Can you work these out from the model? Positions are in its coordinate system, mm. Face numbers are marked on the shaded views. A direction names the side the tool comes from. Coordinates: 2 decimals unless noted, no trailing zeros. Loops run counter-clockwise (first coordinate to the right, second up) from the corner with the lowest first, then second, coordinate; pieces in that order, holes last.
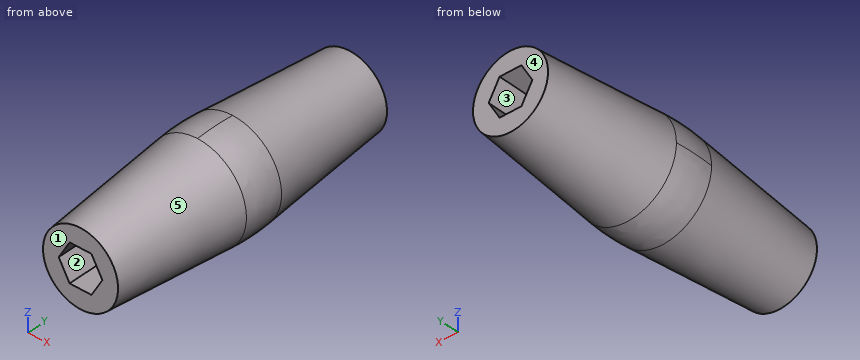
```python
from build123d import *

# Parameters (mm, degrees)
SKETCH1_R           = 12.7
BOSS_EXTRUDE1_DEPTH = 101.6
SKETCH2_R           = 12.7
BOSS_EXTRUDE2_DEPTH = 50.8
BOSS_EXTRUDE2_DRAFT = 5
SKETCH3_R           = 12.7
BOSS_EXTRUDE3_DEPTH = 50.8
BOSS_EXTRUDE3_DRAFT = 5
CUT_EXTRUDE1_DEPTH  = 105.452968153
FILLET2_R           = 76.2


with BuildPart() as part:
    # Sketch1 → Boss-Extrude1 (new body)
    with BuildSketch(Plane(origin=(0, 0, 0), x_dir=(1, 0, 0), z_dir=(0, 1, 0))):
        with Locations(Location((0, 0, 0), (0, 0, 270))):
            Circle(SKETCH1_R)
    extrude(amount=BOSS_EXTRUDE1_DEPTH)


with BuildPart() as boss_extrude2_tool:
    # Sketch2 → Boss-Extrude2 (with draft: the straight prism first)
    with BuildSketch(Plane(origin=(0, 101.6, 0), x_dir=(1, 0, 0), z_dir=(0, 1, 0))):
        with Locations(Location((0, 0, 0), (0, 0, 270))):
            Circle(SKETCH2_R)
    extrude(amount=-BOSS_EXTRUDE2_DEPTH)
    # Boss-Extrude2: the draft: its side faces are tilted about the plane it starts from
    boss_extrude2_sides = [boss_extrude2_tool.faces().sort_by_distance(p)[0] for p in [
        (0, 76.2, -12.7),
    ]]
    draft(boss_extrude2_sides, Plane(origin=(0, 101.6, 0), x_dir=(1, 0, 0), z_dir=(0, 1, 0)), BOSS_EXTRUDE2_DRAFT)


with BuildPart() as part_1:
    add(part.part)

    # Boss-Extrude2: add boss_extrude2_tool
    add(boss_extrude2_tool.part)


with BuildPart() as boss_extrude3_tool:
    # Sketch3 → Boss-Extrude3 (with draft: the straight prism first)
    with BuildSketch(Plane(origin=(0, 0, 0), x_dir=(-1, 0, 0), z_dir=(0, -1, 0))):
        Circle(SKETCH3_R)
    extrude(amount=-BOSS_EXTRUDE3_DEPTH)
    # Boss-Extrude3: the draft: its side faces are tilted about the plane it starts from
    boss_extrude3_sides = [boss_extrude3_tool.faces().sort_by_distance(p)[0] for p in [
        (12.7, 25.4, 0),
    ]]
    draft(boss_extrude3_sides, Plane(origin=(0, 0, 0), x_dir=(-1, 0, 0), z_dir=(0, -1, 0)), BOSS_EXTRUDE3_DRAFT)


with BuildPart() as part_2:
    add(part_1.part)

    # Boss-Extrude3: add boss_extrude3_tool
    add(boss_extrude3_tool.part)

    # Sketch5 → Cut-Extrude1 (cut, through all)
    with BuildSketch(Plane(origin=(0, 0, 0), x_dir=(-1, 0, 0), z_dir=(0, -1, 0))):
        Polygon((-7.391007206, 0), (-3.695503603, -6.4008), (3.695503603, -6.4008), (7.391007206, 0), (3.695503603, 6.4008), (-3.695503603, 6.4008), align=None)
    extrude(amount=-CUT_EXTRUDE1_DEPTH, mode=Mode.SUBTRACT)

    # Fillet2
    fillet2_edges = [part_2.edges().sort_by_distance(p)[0] for p in [
        (12.122938546, 50.8, -12.122938546),
    ]]
    fillet(fillet2_edges, radius=FILLET2_R)


solid = part_2.part
```
(1) I want a section at A-A on y = 81.5. Write out the boundary of the cut face in (x, z), then the cut area to 3 significant figures.
Check values:
outline: circle Ø28.92 at (0, 0); hole (-7.39, 0) - (-3.7, -6.4) - (3.7, -6.4) - (7.39, 0) - (3.7, 6.4) - (-3.7, 6.4) - close
area: 515 mm2
(2) I want a section at B-B on y = 18. Write out the boundary of the cut face in (x, z).
Check values:
outline: circle Ø28.55 at (0, 0); hole (-7.39, 0) - (-3.7, -6.4) - (3.7, -6.4) - (7.39, 0) - (3.7, 6.4) - (-3.7, 6.4) - close
(3) Which directions (+Z, -Z, +X, -X, +Y, -Y) give clear straight access to the entire face, cutting with the end or side of a thin tool? Please do the marked faces 1 and 2.
Check values:
face 1: +Z, -Z, +X, -X, -Y
face 2: +Y, -Y
(4) If I drill on probe 1 along Z at (x, y) = (5, 74); probe 2 along X at (y, z) = (5.5, 0); probe 3 along Z at (x, y) = (-0.5, 69), over which ranges is the centre line in solid material (lowest first)?
Check values:
probe 1: z = -14.26 to -4.14, 4.14 to 14.26
probe 2: x = -13.18 to -7.39, 7.39 to 13.18
probe 3: z = -15.54 to -6.4, 6.4 to 15.54
(5) If we mould it in two halves opening along X, with no side actions, what happens to the marked faces 3, 4 and 5? For each: released by +X, released by -X, zero draft, split by the parting line, or undercut.
Check values:
face 3: undercut
face 4: zero draft
face 5: split by the parting line
(6) I'm going to push flat-ended pins straight in: pin 1 (3.5 mm diameter, centred on x = 0, y = 34.5, fed in from -Z); pin 2 (6 mm diameter, centred on y = 43.5, z = 3.5, fed in from -X); pin 3 (12 mm diameter, centred on x = -9.5, y = 71.5, fed in from -Z). Where does each tip first touch, or does it pass through?
Check values:
pin 1: stops at z = -15.87
pin 2: stops at x = -16.62
pin 3: stops at z = -15.02
